Could you check a few things on this model? Use its own coordinates, in mm. A direction names the side the tool comes from. Coordinates: 2 decimals unless noted, no trailing zeros. Write each loop counter-clockwise with the first axis right and the second up, starting at its lowest first coordinate (ties: lowest second). Pieces come first, ordered by that corner, then holes.
Autodesk Inventor part; units mm, degrees
ref_plane "YZ Plane" through (0, 0, 0) normal (1, 0, 0) x (0, 1, 0)
ref_plane "XZ Plane" through (0, 0, 0) normal (0, 1, 0) x (-1, 0, 0)
ref_plane "XY Plane" through (0, 0, 0) normal (0, 0, 1) x (1, 0, 0)
sketch "Boceto11" plane through (0, 0, 0) normal (0, 1, 0) x (-1, 0, 0)
  line L0 (0, 0) -> (5.6, 0)
  line L1 (5.6, 0) -> (2.8, -4.8497)
  line L2 (2.8, -4.8497) -> (-2.8, -4.8497)
  line L3 (-2.8, -4.8497) -> (-5.6, 0)
  line L4 (-5.6, 0) -> (-2.8, 4.8497)
  line L5 (-2.8, 4.8497) -> (2.8, 4.8497)
  line L6 (2.8, 4.8497) -> (5.6, 0)
  line L7 (5.6, 0) -> (9.1, 0)
  line L8 (9.1, 0) -> (4.55, -7.8808)
  line L9 (4.55, -7.8808) -> (-4.55, -7.8808)
  line L10 (-4.55, -7.8808) -> (-9.1, 0)
  line L11 (-9.1, 0) -> (-4.55, 7.8808)
  line L12 (-4.55, 7.8808) -> (4.55, 7.8808)
  line L13 (4.55, 7.8808) -> (9.1, 0)
  dimension "d42" = 5.6
  dimension "d43" = 3.5
extrude "Extrusión10" add sketch "Boceto11" along normal blind 32
sketch "Boceto16" plane through (0, 0, 0) normal (0, -1, 0) x (1, 0, 0)
  line L0 (4.55, 7.8808) -> (9.1, 0)
  line L1 (9.1, 0) -> (4.55, -7.8808)
  line L2 (4.55, -7.8808) -> (-4.55, -7.8808)
  line L3 (-4.55, -7.8808) -> (-9.1, 0)
  line L4 (-9.1, 0) -> (-4.55, 7.8808)
  line L5 (-4.55, 7.8808) -> (4.55, 7.8808)
  line L6 (4.55, 7.8808) -> (9.1, 0)
  point P0 (0, 0)
  point P1 (0, 0)
extrude "Extrusión14" add sketch "Boceto16" along normal blind 10 draft -23
sketch "Boceto19" plane through (0, -10, 0) normal (0, -1, 0) x (1, 0, 0)
  line L0 (-2.0993, 3.6361) -> (2.0993, 3.6361)
  line L1 (2.0993, -3.6361) -> (-2.0993, -3.6361)
  line L2 (2.0993, 3.6361) -> (4.1986, 0)
  line L3 (-4.55, -7.8808) -> (-2.0993, -3.6361)
  line L4 (-4.1986, 0) -> (-2.0993, 3.6361)
  arc A0 (-1.4491, 2.825) -> (1.4491, 2.825) centre (0, 0) ccw
  line L5 (0, 2.825) -> (-1.4491, 2.825)
  line L6 (0, 2.825) -> (1.4491, 2.825)
extrude "Extrusión16" cut sketch "Boceto19" against normal blind 15
sketch "Boceto20" plane through (0, 0, 0) normal (0, 1, 0) x (1, 0, 0)
  line L0 (-4.55, -7.8808) -> (-2.0993, -3.6361)
  line L1 (-2.7798, -4.8148) -> (-5.5597, 0)
  line L2 (-5.5597, 0) -> (-2.7798, 4.8148)
  line L3 (-2.7798, 4.8148) -> (2.7798, 4.8148)
  line L4 (2.7798, 4.8148) -> (5.5597, 0)
  line L5 (5.5597, 0) -> (2.7798, -4.8148)
  line L6 (2.7798, -4.8148) -> (-2.7798, -4.8148)
  point P0 (0, 0)
  point P1 (0, 0)
extrude "Extrusión17" add sketch "Boceto20" along normal blind 5
sketch "Boceto21" plane through (0, 32, 0) normal (0, 1, 0) x (1, 0, 0)
  line L0 (-2.8, -4.8497) -> (-5.6, 0)
  line L1 (-5.6, 0) -> (-2.8, 4.8497)
  line L2 (-2.8, 4.8497) -> (2.8, 4.8497)
  line L3 (2.8, 4.8497) -> (5.6, 0)
  line L4 (5.6, 0) -> (2.8, -4.8497)
  line L5 (2.8, -4.8497) -> (-2.8, -4.8497)
  line L6 (-2.8, -4.8497) -> (-5.6, 0)
  line L7 (-9, 0) -> (-4.5, 7.7942)
  line L8 (-4.5, 7.7942) -> (4.5, 7.7942)
  line L9 (4.5, 7.7942) -> (9, 0)
  line L10 (9, 0) -> (4.5, -7.7942)
  line L11 (4.5, -7.7942) -> (-4.5, -7.7942)
  line L12 (-4.5, -7.7942) -> (-9, 0)
  point P0 (0, 0)
  point P1 (0, 0)
  point P2 (0, 0)
extrude "Extrusión18" add sketch "Boceto21" along normal blind 5
chamfer "Chaflán1" distance 0.5 angle 45 6 edges at (0, 0, -7.8808) (-6.825, 0, -3.9404) (6.825, 0, -3.9404) (-6.825, 0, 3.9404) (0, 0, 7.8808) (6.825, 0, 3.9404)
properties part number "Bobinatge - acoplament eix"
Item 1: I want a section at C-C, the plane z = 0.75. List the corners of the cut face in (x, y) for me, then the cut area to 3 significant figures.
Item 2: I want a section at B-B, the plane x = 0. List the corners of the cut face in (y, z) for me (3 decimals), then the cut area to 3 significant figures.
Item 3: If we mould it in two halves opening along X, with no side actions, what happens to faces 1 (the flat face through (6.79, 16.03, -4)), 2 (the flat face through (0, 5, 0)), 3 (the flat face through (-0.06, -4.1, 6.14))? For each: released by +X, released by -X, zero draft, split by the parting line, or undercut.
Item 4: Will these pins go through, and if not, where does the flat tip stop? pin 1 Ø1.5 at (y, z) = (7, 4.5) entering from -X; pin 2 Ø6.5 at (x, z) = (-0.5, 1) entering from -Y; pin 3 Ø2.5 at (x, y) = (-0.5, 33.5) entering from +Z; pin 4 Ø8.5 at (x, z) = (0, 0) entering from +Y.
Item 5: I want a section at D-D, the plane y = 13.5. List the corners of the cut face in (x, z) for me, then the cut area to 3 significant figures.
Item 6: Which directions (+Z, -Z, +X, -X, +Y, -Y) give clear straight access to the entire face, cutting with the end or side of a thin tool? Please do faces 4 (the flat face through (0, 16, 7.881)), 5 (the flat face through (-4.22, 18.24, -2.39)), 6 (the cylindrical face through (-0.119, -5.07, -3.173)).
Item 7: I want a section at A-A, the plane y = 34. List the corners of the cut face in (x, z) for me, then the cut area to 3 significant figures.
Item 8: If I drill on line 1 along Z through (x, y) = (2.25, 13.5); line 2 along Y through (x, z) = (-1.5, -0.25); line 3 along X through (y, z) = (11, 2.25), over which ranges is the centre line in solid material (lowest first)?
Taken from the geometry:
1. outline: (-8.67, 0.5) - (-8.44, -0.46) - (-3.77, -10) - (-3.09, -10) - (-3.09, 0) - (3.09, 0) - (3.09, -10) - (3.77, -10) - (8.44, -0.46) - (8.67, 0.5) - (8.67, 32) - (8.57, 32) - (8.57, 37) - (5.17, 37) - (5.17, 0) - (5.13, 0) - (5.13, 5) - (-5.13, 5) - (-5.13, 0) - (-5.17, 0) - (-5.17, 37) - (-8.57, 37) - (-8.57, 32) - (-8.67, 32) - close
1. area: 372 mm2
2. outline: (-10, -3.636) - (-0.46, -7.685) - (0.5, -7.881) - (32, -7.881) - (32, -7.794) - (37, -7.794) - (37, -4.85) - (0, -4.85) - (0, -4.815) - (5, -4.815) - (5, 4.815) - (0, 4.815) - (0, 4.85) - (37, 4.85) - (37, 7.794) - (32, 7.794) - (32, 7.881) - (0.5, 7.881) - (-0.46, 7.685) - (-10, 3.636) - (-10, 2.825) - (0, 2.825) - (0, -3.175) - (-10, -3.175) - close
2. area: 327 mm2
3. face 1: released by +X
3. face 2: undercut
3. face 3: zero draft
4. pin 1: stops at x = -6.93
4. pin 2: stops at y = -10
4. pin 3: stops at z = 7.79
4. pin 4: stops at y = 5
5. outline: (-9.1, 0) - (-4.55, -7.88) - (4.55, -7.88) - (9.1, 0) - (4.55, 7.88) - (-4.55, 7.88) - close; hole (-5.6, 0) - (-2.8, -4.85) - (2.8, -4.85) - (5.6, 0) - (2.8, 4.85) - (-2.8, 4.85) - close
5. area: 134 mm2
6. face 4: +Z, +X, -X, +Y, -Y
6. face 5: +Y
6. face 6: -Y
7. outline: (-9, 0) - (-4.5, -7.79) - (4.5, -7.79) - (9, 0) - (4.5, 7.79) - (-4.5, 7.79) - close; hole (-5.6, 0) - (-2.8, -4.85) - (2.8, -4.85) - (5.6, 0) - (2.8, 4.85) - (-2.8, 4.85) - close
7. area: 129 mm2
8. line 1: z = -7.88 to -4.85, 4.85 to 7.88
8. line 2: y = 0 to 5
8. line 3: x = -7.8 to -4.3, 4.3 to 7.8
